```python
from build123d import *

# Parameters (mm, degrees)
SKETCH1_R           = 4.66725
SKETCH1_R_2         = 3.175
BOSS_EXTRUDE1_DEPTH = 9.525
BOSS_EXTRUDE2_DEPTH = 3.175
BOSS_EXTRUDE3_DEPTH = 3.175
CIRPATTERN1_COUNT   = 24


with BuildPart() as part:
    # Sketch1 → Boss-Extrude1 (new body)
    with BuildSketch(Plane(origin=(0, 0, 0), x_dir=(1, 0, 0), z_dir=(0, 1, 0))):
        Circle(SKETCH1_R)
        Circle(SKETCH1_R_2, mode=Mode.SUBTRACT)
    extrude(amount=BOSS_EXTRUDE1_DEPTH)

    # Sketch2 → Boss-Extrude2 (add)
    with BuildSketch(Plane(origin=(0, 0, 0), x_dir=(1, 0, 0), z_dir=(0, 1, 0))):
        with BuildLine():
            Line((0.635, 5.551803221), (-0.635, 5.551803221))
            ThreePointArc((-0.635, 5.551803221), (-3.720037903, -4.16977961), (5.588, 0))
            ThreePointArc((5.588, 0), (4.16977961, 3.720037903), (0.635, 5.551803221))
        make_face()
    extrude(amount=BOSS_EXTRUDE2_DEPTH)

    # Sketch2_3 → Boss-Extrude3 (add)
    with BuildSketch(Plane(origin=(0, 0, 0), x_dir=(1, 0, 0), z_dir=(0, 1, 0))):
        Polygon((-0.635, 5.551803221), (0.635, 5.551803221), (0.254, 6.858), (-0.254, 6.858), align=None)
    boss_extrude3 = extrude(amount=BOSS_EXTRUDE3_DEPTH)

    # CirPattern1: Boss-Extrude3 ×24 about axis
    cirpattern1_axis = Axis((0, 0, 0), (0, 1, 0))
    for i in range(1, CIRPATTERN1_COUNT):
        add(boss_extrude3.rotate(cirpattern1_axis, i * 360 / CIRPATTERN1_COUNT))


solid = part.part
```
Input: part model. Units: mm. Frame: model coordinates. A direction names the side the tool comes from. Give positions to 0.01 mm unless a question says otherwise; leave off trailing zeros. Loops run counter-clockwise (first coordinate to the right, second up) from the corner with the lowest first, then second, coordinate; pieces in that order, holes last.
1) Reachability of faces 1 (the flat face through (3.485, 1.565, -5.142)), 2 (the flat face through (-6.196, 1.565, -0.447)), 3 (the flat face through (-1.17, 1.57, -6.1)) from +Z, -Z, +X, -X, +Y, -Y: full face, straight path, thin tool, end or side. Return the list, or none.
A:
face 1: +Y, -Y
face 2: -X, +Y, -Y
face 3: -Z, +Y, -Y
2) Mould query, pull axis X, two halves, no side actions, for faces 4 (the flat face through (-0.447, 1.565, 6.196)), 5 (the flat face through (5.6, 1.57, 2.72)), 6 (the flat face through (-6.1, 1.57, 1.17)). Classes: released by +X, released by -X, zero draft, split by the parting line, or undercut.
A:
face 4: undercut
face 5: released by +X
face 6: released by -X
3) Line query: L1, parallel to X at y = 4.75, z = 0 (3 decimals); L2, parallel to Z at x = -6, y = 1.5. Output: solid intervals per line, ascending.
A:
L1: x = -4.667 to -3.175, 3.175 to 4.667
L2: z = -3.32 to -3.14, -2.03 to -1.11, -0.5 to 0.5, 1.11 to 2.03, 3.14 to 3.32
4) Contact query for flat-ended pins moving along their axis: pin 1 (3 mm diameter, centred on x = 3.5, y = 6.5, fed in from +Z); pin 2 (2 mm diameter, centred on x = 4.5, y = 2, fed in from -Z); pin 3 (1.5 mm diameter, centred on x = 5, z = -2, fed in from +Y) (3 decimals); pin 4 (1.9 mm diameter, centred on x = 1.5, z = 1, fed in from +Y) (3 decimals). Output: stop coordinate, or through.
A:
pin 1: stops at z = 4.22
pin 2: stops at z = -5.9
pin 3: stops at y = 9.525
pin 4: stops at y = 3.175
5) Section query B-B on z = 0. Return the cut outline in (x, y) (3 decimals), and give its area (3 significant figures).
A:
outline: (-6.858, 0) - (6.858, 0) - (6.858, 3.175) - (4.667, 3.175) - (4.667, 9.525) - (3.175, 9.525) - (3.175, 3.175) - (-3.175, 3.175) - (-3.175, 9.525) - (-4.667, 9.525) - (-4.667, 3.175) - (-6.858, 3.175) - close
area: 62.5 mm2
6) Section query A-A on x = 0. Return the cut outline in (y, z) (3 decimals), and give its area (3 significant figures).
A:
outline: (0, -6.858) - (3.175, -6.858) - (3.175, -4.667) - (9.525, -4.667) - (9.525, -3.175) - (3.175, -3.175) - (3.175, 3.175) - (9.525, 3.175) - (9.525, 4.667) - (3.175, 4.667) - (3.175, 6.858) - (0, 6.858) - close
area: 62.5 mm2
7) Section query D-D on x = 4. Return the cut outline in (y, z) (3 decimals).
A:
outline: (0, -4.662) - (3.175, -4.662) - (3.175, -2.405) - (9.525, -2.405) - (9.525, 2.405) - (3.175, 2.405) - (3.175, 4.662) - (0, 4.662) - close
